```python
from build123d import *

# Parameters (mm, degrees)
F0_R     = 3.175
F1_DEPTH = 3.048
F2_DEPTH = 25.4


with BuildPart() as f1:
    # F0 (on Top) → F1 (new body)
    with BuildSketch(Plane.XY):
        with BuildLine():
            Line((9.5045213227, 49.566365397), (9.3611481588, 50.7012339615))
            ThreePointArc((9.3611481588, 50.7012339615), (-0.1400603656, 58.4660764801), (-9.4088285736, 50.4252009888))
            Line((-9.4088285736, 50.4252009888), (-9.4825060338, 49.840830011))
            ThreePointArc((-9.4825060338, 49.840830011), (-0.4498638837, 39.4277357171), (9.525, 48.9421062946))
            ThreePointArc((9.525, 48.9421062946), (9.519878954, 49.2544037502), (9.5045213227, 49.566365397))
        make_face()
        with Locations((0, 48.9421062946)):
            Circle(F0_R, mode=Mode.SUBTRACT)
        with BuildLine():
            ThreePointArc((9.5045213227, 49.566365397), (9.4498863967, 50.1359538934), (9.3611481588, 50.7012339615))
            Line((9.3611481588, 50.7012339615), (9.5045213227, 49.566365397))
        make_face()
        with BuildLine():
            Line((-9.4825060338, 49.840830011), (-9.4088285736, 50.4252009888))
            ThreePointArc((-9.4088285736, 50.4252009888), (-9.4501853512, 50.1335851351), (-9.4825060338, 49.840830011))
        make_face()
        with BuildLine():
            Line((15.7498106857, 0.1318520983), (9.5045213227, 49.566365397))
            ThreePointArc((9.5045213227, 49.566365397), (9.519878954, 49.2544037502), (9.525, 48.9421062946))
            ThreePointArc((9.525, 48.9421062946), (-0.4498638837, 39.4277357171), (-9.4825060338, 49.840830011))
            Line((-9.4825060338, 49.840830011), (-15.7503089228, 0.1279043299))
            ThreePointArc((-15.7503089228, 0.1279043299), (-0.0019895424, 14.01710617), (15.7498106857, 0.1318520983))
        make_face()
        with Locations((-3.9544538595, 34.9365547299)):
            Circle(F0_R, mode=Mode.SUBTRACT)
        with BuildLine():
            Line((15.7664681676, 0), (15.7498106857, 0.1318520983))
            ThreePointArc((15.7498106857, 0.1318520983), (15.7581579571, 0.0646262032), (15.7662182853, -0.0026346995))
            Line((15.7662182853, -0.0026346995), (15.7664681676, 0))
        make_face()
        with BuildLine():
            ThreePointArc((15.7662182853, -0.0026346995), (15.7581579571, 0.0646262032), (15.7498106857, 0.1318520983))
            ThreePointArc((15.7498106857, 0.1318520983), (-0.0019895424, 14.01710617), (-15.7503089228, 0.1279043299))
            ThreePointArc((-15.7503089228, 0.1279043299), (-15.7583892955, 0.0627290611), (-15.7661999721, -0.002479078))
            Line((-15.7661999721, -0.002479078), (-15.1362867475, -6.6441708073))
            ThreePointArc((-15.1362867475, -6.6441708073), (7.04938e-05, -17.7328937052), (15.1363292544, -6.64403638))
            Line((15.1363292544, -6.64403638), (15.7662182853, -0.0026346995))
        make_face()
        with Locations((0, -1.8578937054)):
            Circle(F0_R, mode=Mode.SUBTRACT)
        with BuildLine():
            ThreePointArc((-15.7661999721, -0.002479078), (-15.7583892955, 0.0627290611), (-15.7503089228, 0.1279043299))
            Line((-15.7503089228, 0.1279043299), (-15.7664350935, 0))
            Line((-15.7664350935, 0), (-15.7661999721, -0.002479078))
        make_face()
        with BuildLine():
            ThreePointArc((15.875, -1.8578937054), (15.8477812371, -0.9286709871), (15.7662182853, -0.0026346995))
            Line((15.7662182853, -0.0026346995), (15.1363292544, -6.64403638))
            ThreePointArc((15.1363292544, -6.64403638), (15.6892455509, -4.2792980589), (15.875, -1.8578937054))
        make_face()
        with BuildLine():
            Line((-15.1362867475, -6.6441708073), (-15.7661999721, -0.002479078))
            ThreePointArc((-15.7661999721, -0.002479078), (-15.8040798094, -3.356788758), (-15.1362867475, -6.6441708073))
        make_face()
        with BuildLine():
            Line((11.2321620564, -47.8086563632), (15.1363292544, -6.64403638))
            ThreePointArc((15.1363292544, -6.64403638), (7.04938e-05, -17.7328937052), (-15.1362867475, -6.6441708073))
            Line((-15.1362867475, -6.6441708073), (-9.4824478856, -66.257230737))
            ThreePointArc((-9.4824478856, -66.257230737), (-0.4501715725, -55.8435376812), (9.525, -65.3578937054))
            ThreePointArc((9.525, -65.3578937054), (6.9705567315, -71.8491927936), (0.6773435479, -74.8587794913))
            Line((0.6773435479, -74.8587794913), (44.7324052746, -73.2903683199))
            ThreePointArc((44.7324052746, -73.2903683199), (36.5125, -65.3578937054), (44.7324052746, -57.4254190908))
            Line((44.7324052746, -57.4254190908), (18.8639877306, -56.5044734952))
            ThreePointArc((18.8639877306, -56.5044734952), (13.1715436826, -53.8034899802), (11.2321620564, -47.8086563632))
        make_face()
        with BuildLine():
            ThreePointArc((9.525, -65.3578937054), (-0.4501715725, -55.8435376812), (-9.4824478856, -66.257230737))
            ThreePointArc((-9.4824478856, -66.257230737), (-6.4093462917, -72.4038787403), (0, -74.8828937054))
            Line((0, -74.8828937054), (0.6773435479, -74.8587794913))
            ThreePointArc((0.6773435479, -74.8587794913), (6.9705567315, -71.8491927936), (9.525, -65.3578937054))
        make_face()
        with Locations((0, -65.3578937054)):
            Circle(F0_R, mode=Mode.SUBTRACT)
        with BuildLine():
            Line((0.6773435479, -74.8587794913), (0, -74.8828937054))
            ThreePointArc((0, -74.8828937054), (0.3388863295, -74.8768632429), (0.6773435479, -74.8587794913))
        make_face()
        with BuildLine():
            ThreePointArc((52.3875, -65.3578937054), (50.1616327839, -59.8459832206), (44.7324052746, -57.4254190908))
            ThreePointArc((44.7324052746, -57.4254190908), (36.5125, -65.3578937054), (44.7324052746, -73.2903683199))
            ThreePointArc((44.7324052746, -73.2903683199), (50.1616327839, -70.8698041901), (52.3875, -65.3578937054))
        make_face()
        with Locations((44.45, -65.3578937054)):
            Circle(F0_R, mode=Mode.SUBTRACT)
    extrude(amount=F1_DEPTH)

    # F2 (add): a face of the model
    f2_faces = [f1.faces().sort_by_distance(p)[0] for p in [
        (5.2288059098, -18.6652574554, 3.048),
    ]]
    extrude(f2_faces, amount=F2_DEPTH)


solid = f1.part
```
Check sheet for the modelled part. Datum: model origin and axes. Units: mm. Coordinates: 2 decimals unless noted, no trailing zeros. Order: outer loops, then holes, each group sorted by start corner. A loop starts at its lowest first (then second) coordinate and runs counter-clockwise, first axis right, second up. Notation, with made-up numbers: M 50,-38 L 64,-38 A35 cw 64,-1 Z; hole C 86.25,51.5 d7. An arc over 180 degrees is marked long. Write each question's results on one line, items separated by ' | '. Start each with the question number.
1. Mould release check, pull along X, two halves, no side actions. Record for faces 1 (the face through (0.34, 58.46, 14.02)), 2 (the face through (13.157, -27.514, 14.025)), 3 (the face through (-0.688, -68.457, 14.025)), 4 (the face through (-15.81, -3.31, 14.02)): +X half, -X half, draft (parallel to the pull), parting line (faces both ways), or undercut.
2. Cross-section at A-A on z = 3.5. State how many separate pieces and enclosed holes the cut face has, and give its area (3 significant figures).
3. Material ranges on probe 1 along Y at (x, z) = (44.45, 9.25); probe 2 along X at (y, z) = (-1.5, 3.75); probe 3 along X at (y, z) = (46.5, 14.75), recorded low to high.
4. Go/stop test with flat-tipped pins: P1, Ø12, axis at x = 27, z = 14, coming from the -Y side; P2, Ø10, axis at x = 40, z = 12, coming from the +Y side; P3, Ø6, axis at x = 5, z = 12.5, coming from the +Y side. Record where each tip stops, or that it passes through.
5. Cross-section at C-C on y = -49.5. Record the cut outline in (x, z).
6. Cross-section at B-B on x = 23.5. Record the cut outline in (y, z), and give its area (3 significant figures).
Checks:
1) face 1: parting line | face 2: +X half | face 3: undercut | face 4: -X half
2) separate pieces: 1 | enclosed holes: 5 | area: 3,750 mm²
3) probe 1: y = -73.3 to -68.53, -62.18 to -57.42 | probe 2: x = -15.87 to -3.15, 3.15 to 15.87 | probe 3: x = -9.9 to -2.03, 2.03 to 9.89
4) P1: stops at y = -74.14 | P2: stops at y = -57.08 | P3: stops at y = 58.25
5) outline: M -11.07,0 L 11.25,0 L 11.25,28.45 L -11.07,28.45 Z
6) outline: M -74.05,0 L -56.67,0 L -56.67,28.45 L -74.05,28.45 Z | area: 494 mm²
